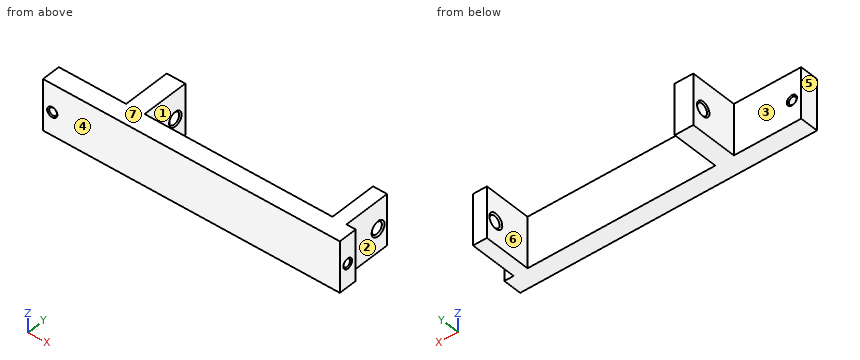
from build123d import *

# Parameters (mm, degrees)
EXTRUDE_1_DEPTH     = 22
M4X0_72_D           = 3.3
M4X0_72_DEPTH       = 11.5
M4X0_72_CSINK_D     = 4.4
M4X0_72_CSINK_ANGLE = 110
M4X0_72_TIP         = 0.991420021


with BuildPart() as part:
    # Эскиз1 → Бобышка-Вытянуть1 (new body)
    with BuildSketch(Plane.XY):
        Polygon((0, 0), (128, 0), (128, 8), (124, 8), (124, 28.5), (118, 28.5), (118, 8), (37, 8), (37, 28.5), (29, 28.5), (29, 8), (0, 8), align=None)
    extrude(amount=EXTRUDE_1_DEPTH)

    # Эскиз2 → Отверстие обработанное метчиком M6x1.01 (revolve, cut)
    with BuildSketch(Plane(origin=(29, 23.5, 10), x_dir=(0, 0, 1), z_dir=(0, 1, 0))):
        Polygon((0, 0), (0, 8), (3.15, 8), (2.5, 7.5448651), (2.5, 0.4551349), (3.15, 0), align=None)
    revolve(axis=Axis((22.65, 23.5, 10), (1, 0, 0)), mode=Mode.SUBTRACT)

    # Эскиз4 → Отверстие обработанное метчиком M6x1.02 (revolve, cut)
    with BuildSketch(Plane(origin=(124, 24, 10), x_dir=(0, 0, -1), z_dir=(0, 1, 0))):
        Polygon((0, 0), (0, 6), (3.25, 6), (2.5, 5.474844346), (2.5, 0.525155654), (3.25, 0), align=None)
    revolve(axis=Axis((130.35, 24, 10), (-1, 0, 0)), mode=Mode.SUBTRACT)

    # Эскиз6 → Отверстие обработанное метчиком M4x0.71 (revolve, cut)
    with BuildSketch(Plane(origin=(4, 0, 10), x_dir=(0, 0, -1), z_dir=(1, 0, 0))):
        Polygon((0, 0), (0, 8), (2.2, 8), (1.65, 7.614885854), (1.65, 0.385114146), (2.2, 0), align=None)
    revolve(axis=Axis((4, -6.35, 10), (0, 1, 0)), mode=Mode.SUBTRACT)

    # Отверстие обработанное метчиком M4x0.72
    with Locations(Plane(origin=(128, 0, 0), x_dir=(0, 0, -1), z_dir=(1, 0, 0))):
        with Locations((-10, 4)):
            CounterSinkHole(M4X0_72_D / 2, M4X0_72_CSINK_D / 2, depth=M4X0_72_DEPTH, counter_sink_angle=M4X0_72_CSINK_ANGLE)
            with Locations((0, 0, -(M4X0_72_DEPTH + M4X0_72_TIP / 2))):  # 118° drill point
                Cone(0, M4X0_72_D / 2, M4X0_72_TIP, mode=Mode.SUBTRACT)


solid = part.part
Could you check a few things on this model? Use its own coordinates, in mm. Face numbers are marked on the shaded views. A direction names the side the tool comes from. Round coordinates to 2 decimals unless told otherwise and drop trailing zeros. Loops run counter-clockwise (first coordinate to the right, second up) from the corner with the lowest first, then second, coordinate; pieces in that order, holes last. Notation, with made-up numbers: (81.5, 87) - (121.5, 87) arc R25 cw to (121.5, 112) - close; hole circle Ø9 at (67, -23). An arc over 180 degrees is marked (long way). Write item = value, one per line.
1) If we mould it in two halves opening along X, with no side actions, what happens to the marked faces 5, 6 and 7? For each: pulls with the +X half, pulls with the -X half, needs draft (parallel to the pull), parting line crosses it, or undercut.
Computed:
face_5 = pulls with the -X half
face_6 = undercut
face_7 = needs draft
2) Imagine slicing it at A-A (y = 10.75). Please give me the cut outline in (x, z).
Computed:
outline = (29, 0) - (37, 0) - (37, 22) - (29, 22) - close; (118, 0) - (124, 0) - (124, 22) - (118, 22) - close
3) On a 3-axis mill with a long thin cutter (end or side, diameter ignored), from which of +Z, -Z, +X, -X, +Y, -Y can I reach the whole of each face in a straight line? I mean the marked faces 1, 2, 3 and 4. Say none if no direction works.
Computed:
face_1 = +Z, -Z, +Y
face_2 = +Z, -Z, +X, +Y
face_3 = +Z, -Z, -X, +Y
face_4 = +Z, -Z, +X, -X, -Y
4) I'm going to push flat-ended pins straight in: P1, Ø6, axis at y = 13.5, z = 11, coming from the -X side; P2, Ø1.5, axis at y = 12, z = 7, coming from the +X side; P3, Ø6.5, axis at x = 12, z = 14.5, coming from the +Y side. Where does each tip first touch, or does it pass through?
Computed:
P1 = 29
P2 = 124
P3 = 8
5) I need wall thicknesses on line 1 along Y through (x, z) = (121.4, 10); line 2 along X through (y, z) = (22.5, 18.25); line 3 along Z through (x, y) = (123.75, 4). Which ranges of each line are inside material? Lowest first, please. Write a range as from..to.
Computed:
line_1 = 0..2.35, 5.65..21.5, 26.5..28.5
line_2 = 29..37, 118..124
line_3 = 0..8.35, 11.65..22
6) Imagine slicing it at C-C (x = 73). Please give me the cut outline in (y, z).
Computed:
outline = (0, 0) - (8, 0) - (8, 22) - (0, 22) - close
7) Imagine slicing it at B-B (z = 17). Please give me the cut outline in (x, y), and give its area (3 significant figures).
Computed:
outline = (0, 0) - (128, 0) - (128, 8) - (124, 8) - (124, 28.5) - (118, 28.5) - (118, 8) - (37, 8) - (37, 28.5) - (29, 28.5) - (29, 8) - (0, 8) - close
area = 1,310 mm2
